from build123d import *

# Parameters (mm, degrees)
F1_DEPTH = 1.6
F2_R     = 3


with BuildPart() as f1:
    # F0 (on Front) → F1 (new body)
    with BuildSketch(Plane.XZ):
        Polygon((-59.5, -68), (58.5, -68), (58.5, -60), (45.5, 0), (45.5, 42), (-45.5, 42), (-45.5, 0), (-59.5, -60), align=None)
    extrude(amount=F1_DEPTH)

    # F2
    f2_edges = [f1.edges().sort_by_distance(p)[0] for p in [
        (-59.5, -0.8, -68),
        (58.5, -0.8, -68),
        (-45.5, -0.8, 42),
        (45.5, -0.8, 42),
        (45.5, -0.8, 0),
        (-45.5, -0.8, 0),
    ]]
    fillet(f2_edges, radius=F2_R)


solid = f1.part
Could you check a few things on this model? Use its own coordinates, in mm. Coordinates: 2 decimals unless noted, no trailing zeros. Loops run counter-clockwise (first coordinate to the right, second up) from the corner with the lowest first, then second, coordinate; pieces in that order, holes last. Notation, with made-up numbers: (9.5, 43.25) -> (35.5, 43.25) arc R13 ccw to (35.5, 53.25) -> close; hole circle Ø6 at (51.25, 8). An arc over 180 degrees is marked (long way). Answer in a Markdown table with one row per item.
(1) Imagine slicing it at B-B (z = -9). List the corners of the cut face in (x, y) for me.
Results found:
| item | result |
|---|---|
| outline | (-47.6, -1.6) -> (47.45, -1.6) -> (47.45, 0) -> (-47.6, 0) -> close |
(2) Will this pin go through, and if not, where does the flat tip stop? pin 1 Ø0.5 at (y, z) = (-0.5, 29) entering from -X.
Results found:
| item | result |
|---|---|
| pin 1 | stops at x = -45.5 |
(3) Imagine slicing it at C-C (x = -49.5). List the corners of the cut face in (y, z) for me, plus the area to 3 significant figures.
Results found:
| item | result |
|---|---|
| outline | (-1.6, -68) -> (0, -68) -> (0, -17.14) -> (-1.6, -17.14) -> close |
| area | 81.4 mm^2 |
(4) If I drill on probe 1 along X at (y, z) = (-1.1, 14); probe 2 along X at (y, z) = (-1.4, -9.5), over which ranges is the centre line in solid material (lowest first)?
Results found:
| item | result |
|---|---|
| probe 1 | x = -45.5 to 45.5 |
| probe 2 | x = -47.72 to 47.56 |
(5) Imagine slicing it at A-A (y = -0.6). List the corners of the cut face in (x, z) for me.
Results found:
| item | result |
|---|---|
| outline | (-59.5, -65) arc R3 ccw to (-56.5, -68) -> (55.5, -68) arc R3 ccw to (58.5, -65) -> (58.5, -60) -> (45.57, -0.31) arc R3 cw to (45.5, 0.32) -> (45.5, 39) arc R3 ccw to (42.5, 42) -> (-42.5, 42) arc R3 ccw to (-45.5, 39) -> (-45.5, 0.35) arc R3 cw to (-45.58, -0.34) -> (-59.5, -60) -> close |
